from build123d import *

# Parameters (mm, degrees)
TROU_TARAUD_M61_D = 5


with BuildPart() as part:
    # Esquisse1 → Révolution1 (revolve)
    with BuildSketch(Plane.XY, mode=Mode.PRIVATE) as r_volution1_sk:
        with BuildLine():
            Line((-0.761813432, 25), (-0.761813432, 49))
            Line((-0.761813432, 49), (-9.761813432, 49))
            Line((-9.761813432, 49), (-23.761813432, 50))
            Line((-23.761813432, 50), (-225.761813432, 50))
            Line((-225.761813432, 50), (-225.761813432, 48.5))
            Line((-225.761813432, 48.5), (-221.761813432, 48.5))
            Line((-221.761813432, 48.5), (-221.761813432, 48))
            Line((-221.761813432, 48), (-214.261813432, 48))
            Line((-214.261813432, 48), (-214.261813432, 45.503048629))
            ThreePointArc((-214.261813432, 45.503048629), (-214.05779592, 45.001981665), (-213.856039491, 44.5))
            Line((-213.856039491, 44.5), (-9.761813432, 44.5))
            Line((-9.761813432, 44.5), (-9.761813432, 15))
            Line((-9.761813432, 15), (-24.761813432, 15))
            Line((-24.761813432, 15), (-24.761813432, 12.5))
            Line((-24.761813432, 12.5), (-64.761813432, 12.5))
            Line((-64.761813432, 12.5), (-64.761813432, 10))
            Line((-64.761813432, 10), (-124.761813432, 10))
            Line((-124.761813432, 10), (-124.761813432, 8.5))
            Line((-124.761813432, 8.5), (-4.761813432, 8.5))
            Line((-4.761813432, 8.5), (-4.761813432, 25))
            Line((-4.761813432, 25), (-0.761813432, 25))
        make_face()
    revolve(r_volution1_sk.sketch.rotate(Axis((0, 0, 0), (-1, 0, 0)), 90), axis=Axis((0, 0, 0), (-1, 0, 0)))

    # Trou taraudé M61 (through all)
    with Locations(Plane(origin=(-0.761813432, 0, 0), x_dir=(0, 0, -1), z_dir=(1, 0, 0))):
        with Locations((40, 10)):
            Hole(TROU_TARAUD_M61_D / 2)


solid = part.part
For this review, take the finished solid that the model builds, in its own axes (mm). A direction names the side the tool comes from. Round coordinates to 2 decimals unless told otherwise and drop trailing zeros. Write each loop counter-clockwise with the first axis right and the second up, starting at its lowest first coordinate (ties: lowest second). Pieces come first, ordered by that corner, then holes. Notation, with made-up numbers: (0.5, 75) - (59.5, 75) arc R8 ccw to (59.5, 79) - close; hole circle Ø3 at (-16, -12.5). An arc over 180 degrees is marked (long way). Write item = value, one per line. Start each with the question number.
1. For pin 1 Ø10 at (x, z) = (-64, -18.5) entering from -Y; pin 2 Ø6 at (x, y) = (-147, -4) entering from +Z; pin 3 Ø25 at (y, z) = (-9, -7) entering from +X, all flat-tipped, find the tip position at first contact; note any pin that passes through.
2. Draft analysis for pull direction Z (two halves, no side actions). For faces 1 (the face through (-225.762, -41, 26.2)), 2 (the face through (-45.042, -3.755, -11.923)), 3 (the face through (-5.325, -14.718, -46.737)), 4 (the face through (-124.762, 7.4, 4.5)), state which applies: released by +Z, released by -Z, zero draft, split by the parting line, or undercut.
3. Consider section B-B on x = -158.5. State the section outline as (y, z) points.
4. Wall thickness on L1, parallel to Y at x = -60, z = 0; L2, parallel to Y at x = -86, z = 0; L3, parallel to Y at x = -45.5, z = -10: over which ranges is each line inside the solid? List them lowest first.
5. Consider section A-A on x = -43. State the section outline as (y, z) points, plus the area to 3 significant figures.
6. For faces 5 (the face through (-63.922, -8.428, 1.107)), 6 (the face through (-221.762, -11, 47)), 7 (the face through (-2.734, -7.509, -23.846)), list the 3-axis set-ups (+Z, -Z, +X, -X, +Y, -Y) from which the entire face can be reached by the end or side of a thin tool; tool diameter is ignored.
7. Consider section C-C on x = -75. State the section outline as (y, z) points.
Evaluation:
q1.pin_1 = -48.14
q1.pin_2 = 49.99
q1.pin_3 = -4.76
q2.face_1 = zero draft
q2.face_2 = undercut
q2.face_3 = split by the parting line
q2.face_4 = undercut
q3.outline = circle Ø100 at (0, 0); hole circle Ø89 at (0, 0)
q4.L1 = -50 to -44.5, -12.5 to -8.5, 8.5 to 12.5, 44.5 to 50
q4.L2 = -50 to -44.5, -10 to -8.5, 8.5 to 10, 44.5 to 50
q4.L3 = -48.99 to -43.36, -7.5 to 7.5, 43.36 to 48.99
q5.outline = circle Ø100 at (0, 0); circle Ø25 at (0, 0); hole circle Ø89 at (0, 0); hole circle Ø17 at (0, 0)
q5.area = 1,900 mm2
q6.face_5 = +X, -X
q6.face_6 = -X
q6.face_7 = +X
q7.outline = circle Ø100 at (0, 0); circle Ø20 at (0, 0); hole circle Ø89 at (0, 0); hole circle Ø17 at (0, 0)
